```python
from build123d import *

# Parameters (mm, degrees)
SKETCH_1_R           = 12
SKETCH_1_R_2         = 1.75
EXTRUDE_1_DEPTH      = 10
SKETCH_2_W           = 110
SKETCH_2_H           = 10
EXTRUDE_2_DEPTH      = 45
SKETCH_5_R           = 3
CUT_EXTRUDE_2_DEPTH  = 91.47651629
SKETCH_6_R           = 5
CUT_EXTRUDE_3_DEPTH  = 5
SKETCH_7_R           = 3
CUT_EXTRUDE_4_DEPTH  = 98.025769773
SKETCH_8_R           = 5
CUT_EXTRUDE_5_DEPTH  = 5
EXTRUDE_3_DEPTH      = 3
EXTRUDE_4_DEPTH      = 3
SKETCH_14_R          = 3
CUT_EXTRUDE_9_DEPTH  = 98.025769773
SKETCH_15_R          = 5
CUT_EXTRUDE_10_DEPTH = 5
SKETCH_16_R          = 3
CUT_EXTRUDE_11_DEPTH = 5


with BuildPart() as part:
    # Эскиз1 → Бобышка-Вытянуть1 (new body)
    with BuildSketch(Plane(origin=(0, 0, 0), x_dir=(1, 0, 0), z_dir=(0, 1, 0))):
        Polygon((-24, 24), (24, 24), (24, -24), (55, -24), (55, -56), (-55, -56), (-55, -24), (-24, -24), align=None)
        with Locations(Location((0, 0, 0), (0, 0, 270))):
            Circle(SKETCH_1_R, mode=Mode.SUBTRACT)
        with Locations(Location((-16, 16, 0), (0, 0, 270))):
            Circle(SKETCH_1_R_2, mode=Mode.SUBTRACT)
        with Locations(Location((16, 16, 0), (0, 0, 270))):
            Circle(SKETCH_1_R_2, mode=Mode.SUBTRACT)
        with Locations(Location((16, -16, 0), (0, 0, 270))):
            Circle(SKETCH_1_R_2, mode=Mode.SUBTRACT)
        with Locations(Location((-16, -16, 0), (0, 0, 270))):
            Circle(SKETCH_1_R_2, mode=Mode.SUBTRACT)
    extrude(amount=EXTRUDE_1_DEPTH)

    # Эскиз2 → Бобышка-Вытянуть2 (add)
    with BuildSketch(Plane(origin=(0, 10, 0), x_dir=(1, 0, 0), z_dir=(0, 1, 0))):
        with Locations((0, -29)):
            Rectangle(SKETCH_2_W, SKETCH_2_H)
    extrude(amount=EXTRUDE_2_DEPTH)

    # Эскиз5 → Вырез-Вытянуть2 (cut, through all)
    with BuildSketch(Plane(origin=(0, 10, 0), x_dir=(1, 0, 0), z_dir=(0, 1, 0))):
        with Locations(Location((-41.25, -44, 0), (0, 0, 270))):
            Circle(SKETCH_5_R)
        with Locations(Location((0, -44, 0), (0, 0, 270))):
            Circle(SKETCH_5_R)
        with Locations(Location((41.25, -44, 0), (0, 0, 270))):
            Circle(SKETCH_5_R)
    extrude(amount=-CUT_EXTRUDE_2_DEPTH, mode=Mode.SUBTRACT)

    # Эскиз6 → Вырез-Вытянуть3 (cut)
    with BuildSketch(Plane.XZ):
        with Locations(Location((-41.25, 44, 0), (0, 0, 270))):
            Circle(SKETCH_6_R)
        with Locations(Location((0, 44, 0), (0, 0, 270))):
            Circle(SKETCH_6_R)
        with Locations(Location((41.25, 44, 0), (0, 0, 270))):
            Circle(SKETCH_6_R)
    extrude(amount=-CUT_EXTRUDE_3_DEPTH, mode=Mode.SUBTRACT)

    # Эскиз7 → Вырез-Вытянуть4 (cut, through all)
    with BuildSketch(Plane.XY.offset(34)):
        with Locations((-41.5, 25)):
            Circle(SKETCH_7_R)
        with Locations((41.5, 25)):
            Circle(SKETCH_7_R)
        with Locations((0, 25)):
            Circle(SKETCH_7_R)
    extrude(amount=-CUT_EXTRUDE_4_DEPTH, mode=Mode.SUBTRACT)

    # Эскиз8 → Вырез-Вытянуть5 (cut)
    with BuildSketch(Plane(origin=(0, 0, 24), x_dir=(-1, 0, 0), z_dir=(0, 0, -1))):
        with Locations((-41.5, 25)):
            Circle(SKETCH_8_R)
        with Locations((0, 25)):
            Circle(SKETCH_8_R)
        with Locations((41.5, 25)):
            Circle(SKETCH_8_R)
    extrude(amount=-CUT_EXTRUDE_5_DEPTH, mode=Mode.SUBTRACT)

    # Эскиз10 → Бобышка-Вытянуть3 (add)
    with BuildSketch(Plane(origin=(24, 0, 0), x_dir=(0, 0, -1), z_dir=(1, 0, 0))):
        Polygon((-24, 10), (-24, 55), (24, 10), align=None)
    extrude(amount=-EXTRUDE_3_DEPTH)

    # Эскиз11 → Бобышка-Вытянуть4 (add)
    with BuildSketch(Plane.ZY.offset(24)):
        Polygon((24, 10), (-24, 10), (24, 55), align=None)
    extrude(amount=-EXTRUDE_4_DEPTH)

    # Эскиз14 → Вырез-Вытянуть9 (cut, through all)
    with BuildSketch(Plane.XY.offset(34)):
        with Locations((-41.5, 47.004834378)):
            Circle(SKETCH_14_R)
        with Locations((41.5, 44.004834378)):
            Circle(SKETCH_14_R)
    extrude(amount=-CUT_EXTRUDE_9_DEPTH, mode=Mode.SUBTRACT)

    # Эскиз15 → Вырез-Вытянуть10 (cut)
    with BuildSketch(Plane(origin=(0, 0, 24), x_dir=(-1, 0, 0), z_dir=(0, 0, -1))):
        with Locations((41.5, 47.004834378)):
            Circle(SKETCH_15_R)
        with Locations((-41.5, 44.004834378)):
            Circle(SKETCH_15_R)
    extrude(amount=-CUT_EXTRUDE_10_DEPTH, mode=Mode.SUBTRACT)

    # Эскиз16 → Вырез-Вытянуть11 (cut)
    with BuildSketch(Plane(origin=(0, 10, 0), x_dir=(1, 0, 0), z_dir=(0, 1, 0))):
        with Locations(Location((16, 16, 0), (0, 0, 270))):
            Circle(SKETCH_16_R)
        with Locations(Location((16, -16, 0), (0, 0, 270))):
            Circle(SKETCH_16_R)
        with Locations(Location((-16, 16, 0), (0, 0, 270))):
            Circle(SKETCH_16_R)
        with Locations(Location((-16, -16, 0), (0, 0, 270))):
            Circle(SKETCH_16_R)
    extrude(amount=-CUT_EXTRUDE_11_DEPTH, mode=Mode.SUBTRACT)


solid = part.part
```
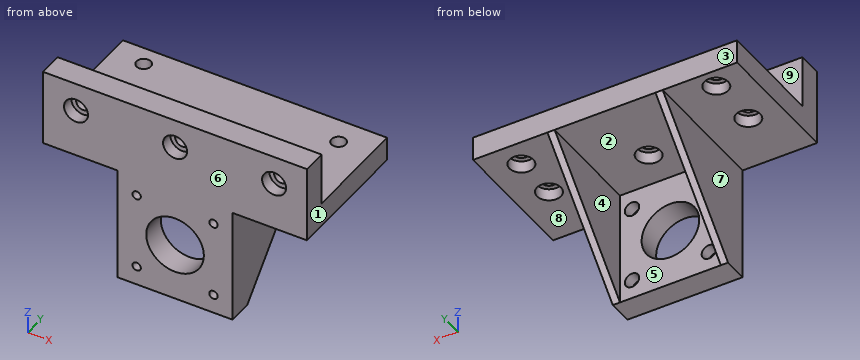
Model file for the job. Use its own axes, mm. Face numbers are marked on the shaded views. A direction names the side the tool comes from. Coordinates: 2 decimals unless noted, no trailing zeros. Write each loop counter-clockwise with the first axis right and the second up, starting at its lowest first coordinate (ties: lowest second). Pieces come first, ordered by that corner, then holes. Notation, with made-up numbers: (-23, 23) - (-14, 23) arc R18 cw to (-14, 54) - close; hole circle Ø8 at (0.25, -2.5). An arc over 180 degrees is marked (long way). One line per question, with ' | ' between items. Start each with the question number.
Q1. Pin check, flat tips, straight feed: pin 1 (5 mm diameter, centred on x = -16, z = -16, fed in from +Y); pin 2 (8 mm diameter, centred on y = 19, z = 0, fed in from +X); pin 3 (7 mm diameter, centred on x = 41.5, y = 44, fed in from -Z); pin 4 (5.5 mm diameter, centred on x = -41.25, z = 44, fed in from -Y). Stop position of each tip, or through.
Q2. Cut at A-A, the plane z = 16. List the corners of the cut face in (x, y), then the cut area to 3 significant figures.
Q3. 3-axis set-ups, long thin cutter, end or side, ignore diameter. For the marked faces 5, 6, 7, 8 and 9: which of +Z, -Z, +X, -X, +Y, -Y reach the whole face in a straight line?
Q4. Cut at C-C, the plane x = -16. List the corners of the cut face in (y, z).
Q5. Cut at D-D, the plane z = 0. List the corners of the cut face in (x, y).
Q6. Drill centre lines: line 1 (X direction, y = 2.5, z = 44); line 2 (X direction, y = 2, z = -16); line 3 (Z direction, x = 16, y = 1). Where is each one in solid material? Low to high. Write a range as [from, to].
Q7. Cut at B-B, the plane y = 3. Give the number of separate pieces and of enclosed holes in the cut face, then the cut area to 3 significant figures.
Q8. Pull direction X, two halves, no side cores. Call the marked faces 1, 2, 3 and 4: pulls with the +X half, pulls with the -X half, needs draft (parallel to the pull), parting line crosses it, or undercut.
Answer below:
1) pin 1: y = 5 | pin 2: x = 24 | pin 3: z = 29 | pin 4: through
2) outline: (-24, 0) - (-17.75, 0) - (-17.75, 5) - (-19, 5) - (-19, 10) - (-21, 10) - (-21, 47.5) - (-24, 47.5) - close; (-14.25, 0) - (14.25, 0) - (14.25, 5) - (13, 5) - (13, 10) - (-13, 10) - (-13, 5) - (-14.25, 5) - close; (17.75, 0) - (24, 0) - (24, 47.5) - (21, 47.5) - (21, 10) - (19, 10) - (19, 5) - (17.75, 5) - close | area: 610 mm^2
3) face 5: -Z, +Y | face 6: +Z, -Z, +X, -X, -Y | face 7: -Z, -X, +Y, -Y | face 8: -Z, +X, +Y, -Y | face 9: +Z, +X, -X, +Y
4) outline: (0, -24) - (10, -24) - (10, -19) - (5, -19) - (5, -17.75) - (0, -17.75) - close; (0, -14.25) - (5, -14.25) - (5, -13) - (10, -13) - (10, 13) - (5, 13) - (5, 14.25) - (0, 14.25) - close; (0, 17.75) - (5, 17.75) - (5, 19) - (10, 19) - (10, 24) - (55, 24) - (55, 34) - (10, 34) - (10, 56) - (0, 56) - close
5) outline: (-24, 0) - (-12, 0) - (-12, 10) - (-21, 10) - (-21, 32.5) - (-24, 32.5) - close; (12, 0) - (24, 0) - (24, 32.5) - (21, 32.5) - (21, 10) - (12, 10) - close
6) line 1: [-55, -46.25], [-36.25, -5], [5, 36.25], [46.25, 55] | line 2: [-24, -17.75], [-14.25, 14.25], [17.75, 24] | line 3: [-24, -17.75], [-14.25, 14.25], [17.75, 56]
7) separate pieces: 1 | enclosed holes: 8 | area: 5,100 mm^2
8) face 1: pulls with the +X half | face 2: undercut | face 3: needs draft | face 4: undercut
